Autodesk Inventor part; units mm, degrees
ref_plane "YZ Plane" through (0, 0, 0) normal (1, 0, 0) x (0, 1, 0)
ref_plane "XZ Plane" through (0, 0, 0) normal (0, 1, 0) x (-1, 0, 0)
ref_plane "XY Plane" through (0, 0, 0) normal (0, 0, 1) x (1, 0, 0)
sketch "Sketch8" plane through (0, 0, 0) normal (0, 1, 0) x (-1, 0, 0)
  line L0 (4.55, 0) -> (-4.55, 0)
  line L1 (-4.55, 0) -> (-4.55, -62.26)
  line L2 (-4.55, -62.26) -> (4.55, -62.26)
  line L3 (4.55, -62.26) -> (4.55, 0)
  point P0 (0, 0)
  point P1 (0, 0)
  dimension "d46" = 62.26
  dimension "pheight" = 9.1
extrude "Extrusion8" add sketch "Sketch8" along normal blind 3.2
sketch "Sketch9" plane through (4.55, 0, -62.26) normal (0, 0, -1) x (-1, 0, 0)
  line L0 (9.1, 0) -> (9.1, 3.2)
  line L1 (0, 0) -> (0, 3.2)
  line L2 (9.1, 1.7) -> (0, 1.7)
  line L3 (0, 1.7) -> (0, 0)
  line L4 (0, 0) -> (9.1, 0)
  line L5 (9.1, 0) -> (9.1, 1.7)
  line L6 (0, 3.2) -> (9.1, 3.2)
  line L7 (0, 0) -> (9.1, 0)
  point P0 (4.55, 0)
  dimension "psnap" = 1.7
  dimension "d65" = 0
extrude "Extrusion9" add sketch "Sketch9" along normal blind 7.24 contours L4 L1 L2 L0
sketch "Sketch10" plane through (-4.55, 0, -62.26) normal (0, 1, 0) x (1, 0, 0)
  line L0 (1.575, 1.93) -> (7.525, 1.93)
  line L1 (7.525, 1.93) -> (7.525, 4.43)
  line L2 (7.525, 4.43) -> (1.575, 4.43)
  line L3 (1.575, 4.43) -> (1.575, 1.93)
  line L4 (0, 7.24) -> (9.1, 7.24)
  line L5 (0, -62.26) -> (0, 7.24)
  line L6 (9.1, -62.26) -> (9.1, 7.24)
  point P0 (4.55, -62.26)
  dimension "phheight" = 5.95
  dimension "phwidth" = 2.5
  dimension "d66" = 2.81
  dimension "d67" = 1.575
  dimension "d68" = 1.575
extrude "Extrusion10" cut sketch "Sketch10" along normal blind 7
equation "\"d68\" = d67"
properties part number "switcher"
Source: CAD feature listing. Evaluate the final solid. Frame: model axes, mm. A direction names the side the tool comes from. Coordinates: 2 decimals unless noted, no trailing zeros. Loops run counter-clockwise (first coordinate to the right, second up) from the corner with the lowest first, then second, coordinate; pieces in that order, holes last. Notation, with made-up numbers: (23.5, 53) -> (32.5, 53) arc R27 cw to (32.5, 70) -> close; hole circle Ø5 at (39, 56.25). An arc over 180 degrees is marked (long way). One line per item, written item: value. Start each with the question number.
Q1. Mould query, pull axis X, two halves, no side actions, for faces 1 (the face through (0, 1, -64.19)), 2 (the face through (0, 1, -66.69)), 3 (the face through (4.55, 2, -34)), 4 (the face through (0, 3.2, -31)). Classes: pulls with the +X half, pulls with the -X half, needs draft (parallel to the pull), parting line crosses it, or undercut.
Q2. Section query D-D, the plane x = 3.75. Return the cut outline in (y, z).
Q3. Section query C-C, the plane y = 1.15. Return the cut outline in (x, z) (3 decimals), and give its area (3 significant figures).
Q4. Section query B-B, the plane x = -0.75. Return the cut outline in (y, z).
Q5. Section query A-A, the plane z = -65. Return the cut outline in (x, y) (3 decimals).
Q6. Contact query for flat-ended pins moving along their axis: P1, Ø1.2, axis at x = -1.5, y = 2.5, coming from the -Z side; P2, Ø0.5, axis at x = -1, y = 0.5, coming from the +Z side. Output: stop coordinate, or through.
Q7. Set-up query: faces 5 (the face through (-2.975, 1, -65)), 6 (the face through (0, 2, -62.26)), 7 (the face through (0, 1, -69.5)). Return all of +Z, -Z, +X, -X, +Y, -Y with unobstructed straight access to the full face (end or side cutting, diameter ignored); none if empty.
Q8. Line query: line 1 along Z through (x, y) = (1.75, 1.15); line 2 along Z through (x, y) = (-2, 2.85). Output: solid intervals per line, ascending.
Results:
1. face 1: undercut
1. face 2: undercut
1. face 3: pulls with the +X half
1. face 4: needs draft
2. outline: (0, -69.5) -> (1.7, -69.5) -> (1.7, -62.26) -> (3.2, -62.26) -> (3.2, 0) -> (0, 0) -> close
3. outline: (-4.55, -69.5) -> (4.55, -69.5) -> (4.55, 0) -> (-4.55, 0) -> close; hole (-2.975, -66.69) -> (2.975, -66.69) -> (2.975, -64.19) -> (-2.975, -64.19) -> close
3. area: 618 mm^2
4. outline: (0, -69.5) -> (1.7, -69.5) -> (1.7, -66.69) -> (0, -66.69) -> close; (0, -64.19) -> (1.7, -64.19) -> (1.7, -62.26) -> (3.2, -62.26) -> (3.2, 0) -> (0, 0) -> close
5. outline: (-4.55, 0) -> (-2.975, 0) -> (-2.975, 1.7) -> (-4.55, 1.7) -> close; (2.975, 0) -> (4.55, 0) -> (4.55, 1.7) -> (2.975, 1.7) -> close
6. P1: z = -62.26
6. P2: z = 0
7. face 5: +Y, -Y
7. face 6: -Z, +X, -X, +Y
7. face 7: -Z, +X, -X, +Y, -Y
8. line 1: -69.5 to -66.69, -64.19 to 0
8. line 2: -62.26 to 0
